The listing builds one solid part. Answer for the finished solid, in the listing's coordinates (mm). Give positions to 0.01 mm unless a question says otherwise; leave off trailing zeros. Order: outer loops, then holes, each group sorted by start corner. A loop starts at its lowest first (then second) coordinate and runs counter-clockwise, first axis right, second up. Notation, with made-up numbers: (43, 19) - (102, 19) arc R11 ccw to (102, 27) - close; hole circle Ø8 at (62, 9.5). An arc over 180 degrees is marked (long way). Answer as a JSON object with one key per item and string values. Group by question number.
Q1. Consider line 1 (X direction, y = 17.5, z = 1.35); line 2 (X direction, y = 20.5, z = 0.8); line 3 (Y direction, x = 93.5, z = 1.5). Determine where each line is inside the solid, lowest interval first.
Q2. A cutting plane is placed at B-B, the plane x = 55.5. Give the vertices of the cut face in (y, z), and give its area (3 significant figures).
Q3. A cutting plane is placed at C-C, the plane y = 24.5. Give the vertices of the cut face in (x, z), and give its area (3 significant figures).
Q4. A cutting plane is placed at A-A, the plane z = 1. Give the vertices of the cut face in (x, y), and give its area (3 significant figures).
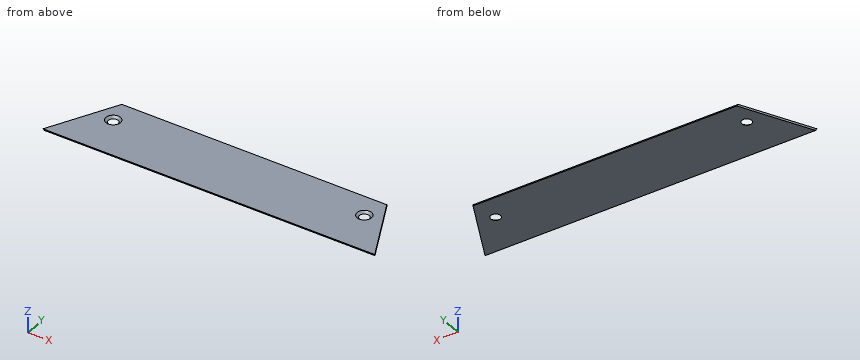
from build123d import *

# Parameters (mm, degrees)
BOSS_EXTRUDE2_DEPTH                       = 162.814
CUT_EXTRUDE1_DEPTH                        = 166.821138692
CSK_FOR_6_FLAT_HEAD_MACHINE_SCREW_2_COUNT = 2
CSK_FOR_6_FLAT_HEAD_MACHINE_SCREW_2_PITCH = 123.248406325


with BuildPart() as part:
    # Sketch3 → Boss-Extrude2 (new body)
    with BuildSketch(Plane(origin=(0, 0, 0), x_dir=(0, 0, -1), z_dir=(1, 0, 0))):
        Polygon((-0.5715, 31.420044321), (-1.5875, 30.833456448), (-1.5875, -1.917455679), (-0.5715, -1.330867805), align=None)
    extrude(amount=BOSS_EXTRUDE2_DEPTH)

    # Sketch5 → Cut-Extrude1 (cut, through all)
    with BuildSketch(Plane.XY.offset(1.5875)):
        Polygon((0, -1.917455679), (16.672349491, 31.420044321), (0, 31.420044321), align=None)
        Polygon((162.814, -1.917455679), (146.141650509, 31.420044321), (162.814, 31.420044321), align=None)
    extrude(amount=-CUT_EXTRUDE1_DEPTH, mode=Mode.SUBTRACT)

    # Sketch7 → CSK for #6 Flat Head Machine Screw (100)1 (revolve, cut)
    with BuildSketch(Plane(origin=(19.939, 19.426957216, 1.5875), x_dir=(0, -1, 0), z_dir=(1, 0, 0))):
        Polygon((0, 0), (0, 1.016), (1.89865, 1.016), (1.89865, 1.380025208), (3.5433, 0), align=None)
    csk_for_6_flat_head_machine_screw_100 = revolve(axis=Axis((19.939, 19.426957216, 7.9375), (0, 0, -1)), mode=Mode.SUBTRACT)

    # CSK for _6 Flat Head Machine Screw _ 2: CSK for #6 Flat Head Machine Screw (100)1 ×2
    with Locations(*[(i * CSK_FOR_6_FLAT_HEAD_MACHINE_SCREW_2_PITCH, 0, 0) for i in range(1, CSK_FOR_6_FLAT_HEAD_MACHINE_SCREW_2_COUNT)]):
        add(csk_for_6_flat_head_machine_screw_100, mode=Mode.SUBTRACT)


solid = part.part
Reply:
{
 "1": {"line 1": "x = 9.71 to 17.31, 22.57 to 140.56, 145.82 to 153.1", "line 2": "x = 11.21 to 17.57, 22.31 to 140.81, 145.56 to 151.6", "line 3": "y = -1.87 to 30.88"},
 "2": {"outline": "(-1.92, 1.59) - (-1.33, 0.57) - (31.42, 0.57) - (30.83, 1.59) - close", "area": "33.3 mm^2"},
 "3": {"outline": "(13.21, 0.57) - (149.6, 0.57) - (149.6, 1.59) - (13.21, 1.59) - close", "area": "139 mm^2"},
 "4": {"outline": "(0.17, -1.58) - (162.64, -1.58) - (146.27, 31.17) - (16.55, 31.17) - close; hole circle Ø5.69 at (19.94, 19.43); hole circle Ø5.69 at (143.19, 19.43)", "area": "4,730 mm^2"}
}
